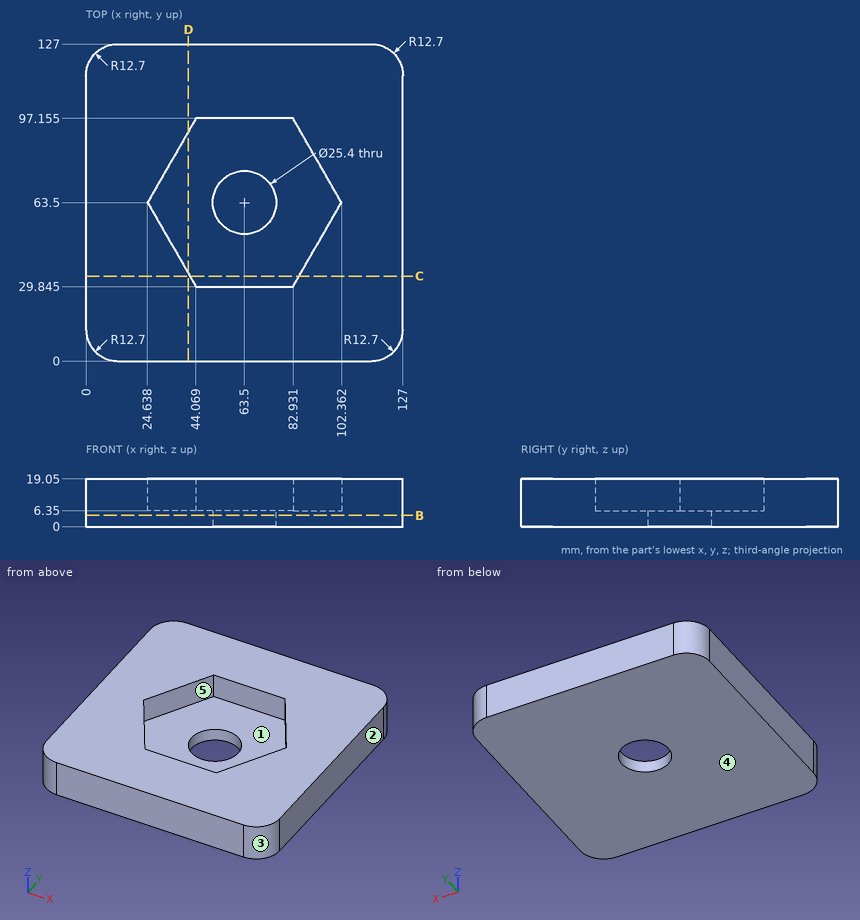
The figure shows three views and two pictorial views of one solid part (mm, origin at its lowest corner). Answer the questions. A direction names the side the tool comes from. Round coordinates to 2 decimals unless told otherwise and drop trailing zeros. Order: outer loops, then holes, each group sorted by start corner. A loop starts at its lowest first (then second) coordinate and runs counter-clockwise, first axis right, second up. Notation, with made-up numbers: M 59,23 L 102,23 A14 ccw 102,46 Z; hole C -18.75,82 d4. An arc over 180 degrees is marked long. Put each result on its own line as item: value. Start each with the question number.
Q1. Straight lines are drawn through the part: L1, parallel to Y at x = 63.5, z = 4.5; L2, parallel to Y at x = 76.5, z = 7.5 (1 decimal). For each, find the intervals that lie inside material, in ascending order. Write a range as [from, to].
Q2. Section C-C, the plane y = 34 is taken. Write down the section's boundary in (x, z).
Q3. Section D-D, the plane x = 41 is taken. Write down the section's boundary in (y, z), and give its area (3 significant figures).
Q4. Section B-B, the plane z = 4.5 is taken. Write down the section's boundary in (x, y), and give its area (3 significant figures).
Q5. For a pull along Y with two mould halves and no side action, classify the marked faces 3, 4 and 5 as pulls with the +Y half, pulls with the -Y half, needs draft (parallel to the pull), parting line crosses it, or undercut.
Q6. A tool of negligible diameter and unlimited length cuts with its end or side. For the marked faces 1 and 2, from which of +Z, -Z, +X, -X, +Y, -Y can it reach the whole face along a straight path? Write none if from no direction.
Findings below:
1. L1: y = [0, 50.8], [76.2, 127]
1. L2: y = [0, 29.8], [97.2, 127]
2. outline: M 0,0 L 127,0 L 127,19.05 L 85.33,19.05 L 85.33,6.35 L 41.67,6.35 L 41.67,19.05 L 0,19.05 Z
3. outline: M 0,0 L 127,0 L 127,19.05 L 91.84,19.05 L 91.84,6.35 L 35.16,6.35 L 35.16,19.05 L 0,19.05 Z
3. area: 1,700 mm^2
4. outline: M 0,12.7 A12.7 ccw 12.7,0 L 114.3,0 A12.7 ccw 127,12.7 L 127,114.3 A12.7 ccw 114.3,127 L 12.7,127 A12.7 ccw 0,114.3 Z; hole C 63.5,63.5 d25.4
4. area: 15,500 mm^2
5. face 3: pulls with the -Y half
5. face 4: needs draft
5. face 5: undercut
6. face 1: +Z
6. face 2: +Z, -Z, +X, +Y, -Y
